The listing builds one solid part. Answer for the finished solid, in the listing's coordinates (mm). Round coordinates to 2 decimals unless told otherwise and drop trailing zeros. Loops run counter-clockwise (first coordinate to the right, second up) from the corner with the lowest first, then second, coordinate; pieces in that order, holes last. Notation, with made-up numbers: (48.25, -2) - (82.25, -2) arc R22 ccw to (82.25, 34) - close; hole circle Ø10 at (59.5, 64). An arc over 180 degrees is marked (long way). One line per question, with ' | ' between items. Start each with the question number.
from build123d import *

# Parameters (mm, degrees)
BOSS_EXTRUDE1_START = 0.15
SKETCH1_W           = 7.4
SKETCH1_H           = 6.8
BOSS_EXTRUDE1_DEPTH = 2.85
FILLET1_R           = 1
CHAMFER1_SIZE       = 1
BOSS_EXTRUDE2_DEPTH = 1.6


with BuildPart() as part:
    # Sketch1 → Boss-Extrude1 (new body)
    with BuildSketch(Plane.XY.offset(BOSS_EXTRUDE1_START)):
        Rectangle(SKETCH1_W, SKETCH1_H)
    extrude(amount=BOSS_EXTRUDE1_DEPTH)

    # Fillet1
    fillet1_edges = [part.edges().sort_by_distance(p)[0] for p in [
        (-3.7, -3.4, 1.575),
        (3.7, 3.4, 1.575),
    ]]
    fillet(fillet1_edges, radius=FILLET1_R)

    # Chamfer1
    chamfer1_edges = [part.edges().sort_by_distance(p)[0] for p in [
        (3.7, -3.4, 1.575),
        (-3.7, 3.4, 1.575),
    ]]
    chamfer(chamfer1_edges, length=CHAMFER1_SIZE)

    # Sketch2 → Boss-Extrude2 (add, symmetric)
    with BuildSketch(Plane(origin=(0, 0, 0), x_dir=(1, 0, 0), z_dir=(0, 1, 0))):
        Polygon((2, -0.15), (3.7, -0.15), (3.7, -2.9), (3.85, -2.9), (3.85, 0), (2, 0), align=None)
    boss_extrude2 = extrude(amount=BOSS_EXTRUDE2_DEPTH, both=True)

    # Mirror1: Boss-Extrude2 across plane
    add(boss_extrude2.mirror(Plane(origin=(0, 0, 0), x_dir=(0, 0, 1), z_dir=(1, 0, 0))))


solid = part.part
(1) Find section C-C on x = 3. Write down the section's boundary in (y, z), plus the area to 3 significant figures.
(2) Find section A-A on z = 2.45. Write down the section's boundary in (x, y).
(3) Consider L1, parallel to X at y = -1.75, z = 1.2; L2, parallel to Z at x = 3.75, y = 1.25; L3, parallel to Z at x = 0.25, y = 0.5. Determine where each line is inside the solid, lowest interval first.
(4) Determine the mould class of faces 1 (the flat face through (0, 3.4, 2)), 2 (the flat face through (0, 0, 0.15)), 3 (the cylindrical face through (-3.415, -3.099, 1.595)) for opening direction X: pulls with the +X half, pulls with the -X half, needs draft (parallel to the pull), parting line crosses it, or undercut.
(5) Find section B-B on y = -1. Write down the section's boundary in (x, z).
(6) Each of these flat-tipped pins is pushed along its axis until it touches: P1, Ø1.5, axis at y = 2.5, z = 0.5, coming from the -X side; P2, Ø2, axis at x = 0.5, y = -0.5, coming from the -Z side. Where does it stop, or does it pass through?
(7) Find section D-D on y = -1.75. Write down the section's boundary in (x, z), plus the area to 3 significant figures.
Answer below:
1) outline: (-3.1, 0.15) - (-1.6, 0.15) - (-1.6, 0) - (1.6, 0) - (1.6, 0.15) - (3.35, 0.15) - (3.35, 3) - (-3.1, 3) - close | area: 18.9 mm2
2) outline: (-3.85, -1.6) - (-3.7, -1.6) - (-3.7, -2.4) arc R1 ccw to (-2.7, -3.4) - (2.7, -3.4) - (3.7, -2.4) - (3.7, -1.6) - (3.85, -1.6) - (3.85, 1.6) - (3.7, 1.6) - (3.7, 2.4) arc R1 ccw to (2.7, 3.4) - (-2.7, 3.4) - (-3.7, 2.4) - (-3.7, 1.6) - (-3.85, 1.6) - close
3) L1: -3.7 to 3.7 | L2: 0 to 2.9 | L3: 0.15 to 3
4) face 1: needs draft | face 2: undercut | face 3: pulls with the -X half
5) outline: (-3.85, 0) - (-2, 0) - (-2, 0.15) - (2, 0.15) - (2, 0) - (3.85, 0) - (3.85, 2.9) - (3.7, 2.9) - (3.7, 3) - (-3.7, 3) - (-3.7, 2.9) - (-3.85, 2.9) - close
6) P1: x = -3.7 | P2: z = 0.15
7) outline: (-3.7, 0.15) - (3.7, 0.15) - (3.7, 3) - (-3.7, 3) - close | area: 21.1 mm2
